Input: part model. Units: mm. Frame: model coordinates. A direction names the side the tool comes from. Coordinates: 2 decimals unless noted, no trailing zeros. Order: outer loops, then holes, each group sorted by start corner. A loop starts at its lowest first (then second) coordinate and runs counter-clockwise, first axis right, second up. Notation, with made-up numbers: (9.25, 9.25) - (45.25, 9.25) arc R8 cw to (45.25, 21.25) - close; hole circle Ø7 at (86.25, 27). An arc over 180 degrees is marked (long way). One line per question, with ' | ' between items.
from build123d import *

# Parameters (mm, degrees)
SKETCH1_W                  = 70.104
SKETCH1_H                  = 38.1
RECTANGULAR_BASE_DEPTH     = 3.175
SKETCH2_R                  = 34.29
CIRCULAR_BASE_ADD_ON_DEPTH = 3.175
SKETCH4_W                  = 3.2258
SKETCH4_H                  = 6.35
TAB_DEPTH                  = 3.175
SKETCH5_R                  = 10.795
CUT_EXTRUDE1_DEPTH         = 4.175
SKETCH6_R                  = 3.4925
CUT_FOR_SCREW_ACCESS_DEPTH = 4.175


with BuildPart() as part:
    # Sketch1 → rectangular base (new body)
    with BuildSketch(Plane(origin=(0, 0, 0), x_dir=(1, 0, 0), z_dir=(0, 1, 0))):
        Rectangle(SKETCH1_W, SKETCH1_H)
    extrude(amount=RECTANGULAR_BASE_DEPTH)

    # Sketch2 → circular base add on (add)
    with BuildSketch(Plane(origin=(0, 3.175, 0), x_dir=(1, 0, 0), z_dir=(0, 1, 0))):
        Circle(SKETCH2_R)
    extrude(amount=-CIRCULAR_BASE_ADD_ON_DEPTH)

    # Sketch4 → tab (add)
    with BuildSketch(Plane(origin=(0, 3.175, 0), x_dir=(1, 0, 0), z_dir=(0, 1, 0))):
        with Locations((-36.6649, 10.795)):
            Rectangle(SKETCH4_W, SKETCH4_H)
        with Locations((-36.6649, -10.795)):
            Rectangle(SKETCH4_W, SKETCH4_H)
    tab = extrude(amount=-TAB_DEPTH)

    # Mirror1: tab across plane
    add(tab.mirror(Plane(origin=(0, 0, 0), x_dir=(0, 0, 1), z_dir=(1, 0, 0))))

    # Sketch5 → Cut-Extrude1 (cut, through all)
    with BuildSketch(Plane(origin=(0, 3.175, 0), x_dir=(1, 0, 0), z_dir=(0, 1, 0))):
        Circle(SKETCH5_R)
    extrude(amount=-CUT_EXTRUDE1_DEPTH, mode=Mode.SUBTRACT)

    # Sketch6 → cut for screw access (cut, through all)
    with BuildSketch(Plane(origin=(0, 3.175, 0), x_dir=(1, 0, 0), z_dir=(0, 1, 0))):
        with Locations((4.955, 15.24)):
            Circle(SKETCH6_R)
        with Locations((-4.955, 15.24)):
            Circle(SKETCH6_R)
    extrude(amount=-CUT_FOR_SCREW_ACCESS_DEPTH, mode=Mode.SUBTRACT)


solid = part.part
Item 1: Section D-D on z = 0. Return the cut outline in (x, y) (3 decimals), and give its area (3 significant figures).
Data:
outline: (-35.052, 0) - (-10.795, 0) - (-10.795, 3.175) - (-35.052, 3.175) - close; (10.795, 0) - (35.052, 0) - (35.052, 3.175) - (10.795, 3.175) - close | area: 154 mm^2
Item 2: Contact query for flat-ended pins moving along their axis: P1, Ø1, axis at x = -31, y = 2, coming from the +Z side; P2, Ø1.6, axis at y = 1.5, z = 16.5, coming from the -X side; P3, Ø1, axis at x = -37.5, y = 1, coming from the +Z side. Output: stop coordinate, or through.
Data:
P1: z = 19.05 | P2: x = -35.05 | P3: z = 13.97
Item 3: Section C-C on x = 0. Return the cut outline in (y, z) (3 decimals), and give its area (3 significant figures).
Data:
outline: (0, -34.29) - (3.175, -34.29) - (3.175, -10.795) - (0, -10.795) - close; (0, 10.795) - (3.175, 10.795) - (3.175, 34.29) - (0, 34.29) - close | area: 149 mm^2
Item 4: Ray query, line 1 (X direction, y = 2.3, z = -15.24); line 2 (X direction, y = 1.5, z = 0) (3 decimals); line 3 (Z direction, x = 6.5, y = 0.6). Return the intervals inside material, ascending.
Data:
line 1: -35.05 to -8.45, -1.46 to 1.46, 8.45 to 35.05 | line 2: -35.052 to -10.795, 10.795 to 35.052 | line 3: -33.67 to -18.37, -12.11 to -8.62, 8.62 to 33.67
Item 5: Access query for faces 1 (the face through (37, 2, 7.62)), 2 (the face through (-32, 2, 19.05)), 3 (the face through (35.052, 2, 17)). Directions: +Z, -Z, +X, -X, +Y, -Y. A direction counts if a zero-diameter tool reaches every point of the face in a straight line with its end or side. Return the directions, or none.
Data:
face 1: +X, +Y, -Y | face 2: +Z, -X, +Y, -Y | face 3: +Z, +X, +Y, -Y
Item 6: Section A-A on y = 1.4. Count the separate pieces of the cut face and the enclosed holes in it, and give its area (3 significant figures).
Data:
separate pieces: 1 | enclosed holes: 3 | area: 3,530 mm^2
Item 7: Section B-B on z = -15.24. Return the cut outline in (x, y) (1 decimal), and give its area (3 significant figures).
Data:
outline: (-35.1, 0) - (-8.4, 0) - (-8.4, 3.2) - (-35.1, 3.2) - close; (-1.5, 0) - (1.5, 0) - (1.5, 3.2) - (-1.5, 3.2) - close; (8.4, 0) - (35.1, 0) - (35.1, 3.2) - (8.4, 3.2) - close | area: 178 mm^2
Item 8: Draft query along Z for faces 4 (the face through (35.052, 2, 0)), 5 (the face through (-38.278, 2, -11)), 6 (the face through (37, 2, -13.97)). Return one class per face: released by +Z, released by -Z, zero draft, split by the parting line, or undercut.
Data:
face 4: undercut | face 5: zero draft | face 6: released by -Z
